```python
from build123d import *

# Parameters (mm, degrees)
F0_W     = 10
F0_H     = 138
F0_W_2   = 4.6593984449
F0_H_2   = 28.3
F0_W_3   = 4.6
F1_DEPTH = 11.95
F2_DEPTH = 9
F4_W     = 10
F4_H     = 138
F4_W_2   = 4.6593984449
F4_H_2   = 28.3
F4_W_3   = 4.6
F5_DEPTH = 6
F6_DEPTH = 7.6


with BuildPart() as f1:
    # F0 (on Front) → F1 (new body)
    with BuildSketch(Plane.XZ):
        with Locations((-25.2545091997, -12.3230710179)):
            Rectangle(F0_W, F0_H)
        with Locations((-25.2918084222, -60.6730710179)):
            Rectangle(F0_W_2, F0_H_2, mode=Mode.SUBTRACT)
        Polygon((-27.5621091997, -41.1834381521), (-27.5621091997, -14.3230710179), (-22.9621091997, -14.3230710179), (-22.9621091997, -42.6230710179), (-27.5621091997, -42.6230710179), align=None, mode=Mode.SUBTRACT)
        with Locations((-25.2621091997, 3.7269289821)):
            Rectangle(F0_W_3, F0_H_2, mode=Mode.SUBTRACT)
        with Locations((-25.2621091997, 35.9269289821)):
            Rectangle(F0_W_3, F0_H_2, mode=Mode.SUBTRACT)
        with Locations((-25.2621091997, 35.9269289821)):
            Rectangle(F0_W_3, F0_H_2)
        with Locations((-25.2621091997, 3.7269289821)):
            Rectangle(F0_W_3, F0_H_2)
        Polygon((-22.9621091997, -14.3230710179), (-27.5621091997, -14.3230710179), (-27.5621091997, -41.1834381521), (-27.5621091997, -42.6230710179), (-22.9621091997, -42.6230710179), align=None)
        with Locations((-25.2918084222, -60.6730710179)):
            Rectangle(F0_W_2, F0_H_2)
    extrude(amount=F1_DEPTH)

    # F0 (on Front) → F2 (cut)
    with BuildSketch(Plane.XZ):
        with Locations((-25.2621091997, 35.9269289821)):
            Rectangle(F0_W_3, F0_H_2)
        with Locations((-25.2621091997, 3.7269289821)):
            Rectangle(F0_W_3, F0_H_2)
        Polygon((-22.9621091997, -14.3230710179), (-27.5621091997, -14.3230710179), (-27.5621091997, -41.1834381521), (-27.5621091997, -42.6230710179), (-22.9621091997, -42.6230710179), align=None)
        with Locations((-25.2918084222, -60.6730710179)):
            Rectangle(F0_W_2, F0_H_2)
    extrude(amount=F2_DEPTH, mode=Mode.SUBTRACT)

    # F3: F1 across face


with BuildPart() as f1_1:
    add(f1.part)
    add(f1.part.mirror(Plane(origin=(-25.2545091997, -11.95, -12.3230710179), x_dir=(1, 0, 0), z_dir=(0, -1, 0))))

    # F4 (on face) → F5 (join)
    with BuildSketch(Plane.YZ.offset(-20.2545091997)):
        with Locations((-11.9253657708, -12.4240700761)):
            Rectangle(F4_W, F4_H)
        with Locations((-11.9626649932, -60.7740700761)):
            Rectangle(F4_W_2, F4_H_2, mode=Mode.SUBTRACT)
        with Locations((-11.9329657708, -28.5740700761)):
            Rectangle(F4_W_3, F4_H_2, mode=Mode.SUBTRACT)
        with Locations((-11.9329657708, 3.6259299239)):
            Rectangle(F4_W_3, F4_H_2, mode=Mode.SUBTRACT)
        with Locations((-11.9329657708, 35.8259299239)):
            Rectangle(F4_W_3, F4_H_2, mode=Mode.SUBTRACT)
    extrude(amount=F5_DEPTH)

    # F6 (cut): faces of the model
    f6_faces = [f1_1.faces().sort_by_distance(p)[0] for p in [
        (-20.2545091997, -11.9329657708, 35.8259299239),
        (-20.2545091997, -11.9329657708, 3.6259299239),
        (-20.2545091997, -11.9329657708, -28.5740700761),
        (-20.2545091997, -11.9626649932, -60.7740700761),
    ]]
    extrude(f6_faces, amount=-F6_DEPTH, mode=Mode.SUBTRACT)


solid = f1_1.part
```
Check sheet for the modelled part. Datum: model origin and axes. Units: mm. A direction names the side the tool comes from. Give positions to 0.01 mm unless a question says otherwise; leave off trailing zeros. Loops run counter-clockwise (first coordinate to the right, second up) from the corner with the lowest first, then second, coordinate; pieces in that order, holes last. Notation, with made-up numbers: M 88,78 L 108,78 A18 ccw 108,82 Z; hole C 38.25,59.25 d10. An arc over 180 degrees is marked long. Answer in a Markdown table with one row per item.
1) Mould release check, pull along Z, two halves, no side actions. Record for faces 1 (the face through (-17, -6.925, -13)), 2 (the face through (-21, -14.292, -61)), 3 (the face through (-17, -12, -81.424)): released by +Z, released by -Z, zero draft, split by the parting line, or undercut.
Solutions:
| item | result |
|---|---|
| face 1 | zero draft |
| face 2 | undercut |
| face 3 | released by -Z |
2) Cross-section at C-C (z = -48). Enter the section's corners in (x, y).
Solutions:
| item | result |
|---|---|
| outline | M -30.25,-23.9 L -27.62,-23.9 L -27.62,-14.9 L -22.96,-14.9 L -22.96,-23.9 L -20.25,-23.9 L -20.25,-16.93 L -14.25,-16.93 L -14.25,-14.29 L -27.85,-14.29 L -27.85,-9.63 L -14.25,-9.63 L -14.25,-6.93 L -20.25,-6.93 L -20.25,0 L -22.96,0 L -22.96,-9 L -27.62,-9 L -27.62,0 L -30.25,0 Z |
3) Cross-section at D-D (z = -2.5). Enter the section's corners in (x, y).
Solutions:
| item | result |
|---|---|
| outline | M -30.25,-23.9 L -27.56,-23.9 L -27.56,-14.9 L -22.96,-14.9 L -22.96,-23.9 L -20.25,-23.9 L -20.25,-16.93 L -14.25,-16.93 L -14.25,-14.23 L -27.85,-14.23 L -27.85,-9.63 L -14.25,-9.63 L -14.25,-6.93 L -20.25,-6.93 L -20.25,0 L -22.96,0 L -22.96,-9 L -27.56,-9 L -27.56,0 L -30.25,0 Z |
4) Thickness scan on line 1 (Z direction, x = -20, y = -11.5); line 2 (Y direction, x = -19, z = -54); line 3 (X direction, y = -19.25, z = -40.5). Record the ranges inside material, lowest first.
Solutions:
| item | result |
|---|---|
| line 1 | z = -81.42 to -74.92, -46.62 to -42.72, -14.42 to -10.52, 17.78 to 21.68, 49.98 to 56.58 |
| line 2 | y = -16.93 to -14.29, -9.63 to -6.93 |
| line 3 | x = -30.25 to -27.56, -22.96 to -20.25 |
5) Depth check by flat-ended pin: pin 1 (2 mm diameter, centred on x = -17, y = -6, fed in from +Z); pin 2 (2.5 mm diameter, centred on x = -22.5, y = -12.5, fed in from -Z); pin 3 (1.4 mm diameter, centred on x = -25, z = -66.5, fed in from -Y). Enter the tip coordinate at first touch or a pass-through.
Solutions:
| item | result |
|---|---|
| pin 1 | stops at z = 56.58 |
| pin 2 | stops at z = -81.32 |
| pin 3 | stops at y = -14.9 |
6) Tool access check on faces 4 (the face through (-25, -4, 50.077)), 5 (the face through (-21, -9.633, 3)), 6 (the face through (-22.962, -19, -29)). Record the directions out of +Z, -Z, +X, -X, +Y, -Y that give a thin tool (end or side, any length) a straight path to the whole face; none if there is none.
Solutions:
| item | result |
|---|---|
| face 4 | +Y |
| face 5 | +X |
| face 6 | -Y |
7) Cross-section at A-A (x = -17). Enter the section's corners in (y, z).
Solutions:
| item | result |
|---|---|
| outline | M -16.93,-81.42 L -6.93,-81.42 L -6.93,56.58 L -16.93,56.58 Z; hole M -14.29,-74.92 L -9.63,-74.92 L -9.63,-46.62 L -14.29,-46.62 Z; hole M -14.23,-42.72 L -9.63,-42.72 L -9.63,-14.42 L -14.23,-14.42 Z; hole M -14.23,-10.52 L -9.63,-10.52 L -9.63,17.78 L -14.23,17.78 Z; hole M -14.23,21.68 L -9.63,21.68 L -9.63,49.98 L -14.23,49.98 Z |
8) Cross-section at B-B (y = -21.75). Enter the section's corners in (x, z).
Solutions:
| item | result |
|---|---|
| outline | M -30.25,-81.32 L -20.25,-81.32 L -20.25,56.68 L -30.25,56.68 Z; hole M -27.62,-74.82 L -22.96,-74.82 L -22.96,-46.52 L -27.62,-46.52 Z; hole M -27.56,-42.62 L -22.96,-42.62 L -22.96,-14.32 L -27.56,-14.32 Z; hole M -27.56,-10.42 L -22.96,-10.42 L -22.96,17.88 L -27.56,17.88 Z; hole M -27.56,21.78 L -22.96,21.78 L -22.96,50.08 L -27.56,50.08 Z |
